Geometry check sheet. Reference: the model listing, model coordinates, mm. Round coordinates to 2 decimals unless told otherwise and drop trailing zeros. Loops run counter-clockwise (first coordinate to the right, second up) from the corner with the lowest first, then second, coordinate; pieces in that order, holes last.
Solid Edge part; units mm, degrees
sketch "Sketch1" plane through (0, 0, 0) normal (1, 0, 0) x (0, 1, 0)
  circle A0 centre (0, 0) radius 5
extrude "Protrusion1" add sketch "Sketch1" along normal mid plane 55
cosmetic_thread "Thread_2" thread depth 15
cosmetic_thread "Thread_3" thread depth 15
hole "Hole_1" at (23.5, -5, 0) direction (0, 1, 0) diameter 2.5 end up to next
hole "Hole1" at (-23.5, -5, 0) direction (0, 1, 0) diameter 2.5 end up to next
1) Mould release check, pull along Z, two halves, no side actions. Record for faces 1 (the face through (22.28, -0.07, 0.27)), 2 (the face through (-0.385, 4.619, 1.915)), 3 (the face through (-27.5, 0, 0)), 4 (the face through (-24.72, -0.07, 0.27)): +Z half, -Z half, draft (parallel to the pull), parting line (faces both ways), or undercut.
Report:
face 1: undercut
face 2: parting line
face 3: draft
face 4: undercut
2) Sectioned sample at A-A, the plane y = 0. Record the cut outline in (x, z).
Report:
outline: (-27.5, -5) - (27.5, -5) - (27.5, 5) - (-27.5, 5) - close; hole circle Ø2.5 at (-23.5, 0); hole circle Ø2.5 at (23.5, 0)
3) Sectioned sample at B-B, the plane z = 4. Record the cut outline in (x, y), then the cut area to 3 significant figures.
Report:
outline: (-27.5, -3) - (27.5, -3) - (27.5, 3) - (-27.5, 3) - close
area: 330 mm2
4) Sectioned sample at D-D, the plane x = -5. Record the cut outline in (y, z).
Report:
outline: circle Ø10 at (0, 0)
5) Scan lines: line 1 along X through (y, z) = (2, 0); line 2 along X through (y, z) = (2.5, -0.5); line 3 along Z through (x, y) = (-23.5, -0.25). Record each from-to range of solid material in increasing order.
Report:
line 1: x = -27.5 to -24.75, -22.25 to 22.25, 24.75 to 27.5
line 2: x = -27.5 to -24.65, -22.35 to 22.35, 24.65 to 27.5
line 3: z = -4.99 to -1.25, 1.25 to 4.99
6) Sectioned sample at C-C, the plane x = -23.5. Record the cut outline in (y, z).
Report:
outline: (-4.84, -1.25) arc R5 ccw to (4.84, -1.25) - close; (-4.84, 1.25) - (4.84, 1.25) arc R5 ccw to start
7) Gauge pin test, flat ends, axial feed: pin 1 (2 mm diameter, centred on x = 5.5, y = 2.5, fed in from -Z); pin 2 (4 mm diameter, centred on x = 5.5, z = -3, fed in from +Y); pin 3 (1.5 mm diameter, centred on x = -21, y = -3.5, fed in from +Z). Record the tip position at first contact, or that the pin passes through.
Report:
pin 1: stops at z = -4.77
pin 2: stops at y = 4.9
pin 3: stops at z = 4.18
